```python
from build123d import *

# Parameters (mm, degrees)
F0_R     = 76.2
F0_R_2   = 1.778
F1_DEPTH = 2.921


with BuildPart() as f1:
    # F0 (on Top) → F1 (new body)
    with BuildSketch(Plane.XY):
        with Locations((76.2, 76.2)):
            Circle(F0_R)
        with Locations((35.250032, 35.250032)):
            Circle(F0_R_2, mode=Mode.SUBTRACT)
        with Locations((76.2, 8.89)):
            Circle(F0_R_2, mode=Mode.SUBTRACT)
        with Locations((117.149968, 35.250032)):
            Circle(F0_R_2, mode=Mode.SUBTRACT)
        with Locations((76.2, 66.675)):
            Circle(F0_R_2, mode=Mode.SUBTRACT)
        with Locations((8.89, 76.2)):
            Circle(F0_R_2, mode=Mode.SUBTRACT)
        with Locations((66.675, 76.2)):
            Circle(F0_R_2, mode=Mode.SUBTRACT)
        with Locations((35.250032, 117.149968)):
            Circle(F0_R_2, mode=Mode.SUBTRACT)
        with Locations((85.725, 76.2)):
            Circle(F0_R_2, mode=Mode.SUBTRACT)
        with Locations((76.2, 85.725)):
            Circle(F0_R_2, mode=Mode.SUBTRACT)
        with Locations((143.51, 76.2)):
            Circle(F0_R_2, mode=Mode.SUBTRACT)
        with Locations((76.2, 143.51)):
            Circle(F0_R_2, mode=Mode.SUBTRACT)
        with Locations((117.149968, 117.149968)):
            Circle(F0_R_2, mode=Mode.SUBTRACT)
    extrude(amount=F1_DEPTH)


solid = f1.part
```
Input: part model. Units: mm. Frame: model coordinates. Coordinates: 2 decimals unless noted, no trailing zeros. Order: outer loops, then holes, each group sorted by start corner. A loop starts at its lowest first (then second) coordinate and runs counter-clockwise, first axis right, second up. Notation, with made-up numbers: (18, 44) - (28, 44) arc R25 ccw to (28, 61) - close; hole circle Ø1 at (35.5, -6.5). An arc over 180 degrees is marked (long way). Put each result on its own line as item: value.
1. Cut plane D-D on z = 1.8. State how many separate pieces and enclosed holes the cut face has, then the cut area to 3 significant figures.
Report:
separate pieces: 1
enclosed holes: 12
area: 18,100 mm2
2. Draft query along Y for faces 1 (the face through (118.846, 35.784, 1.44)), 2 (the face through (66.28, 151.75, 1.44)), 3 (the face through (75, 77, 2.921)). Return one class per face: pulls with the +Y half, pulls with the -Y half, needs draft (parallel to the pull), parting line crosses it, or undercut.
Report:
face 1: undercut
face 2: parting line crosses it
face 3: needs draft
3. Line query: line 1 along Y through (x, z) = (76.2, 1.45); line 2 along X through (y, z) = (34, 2.4); line 3 along Y through (x, z) = (8.89, 1.95). Output: solid intervals per line, ascending.
Report:
line 1: y = 0 to 7.11, 10.67 to 64.9, 68.45 to 83.95, 87.5 to 141.73, 145.29 to 152.4
line 2: x = 12.75 to 33.99, 36.51 to 115.89, 118.41 to 139.65
line 3: y = 40.48 to 74.42, 77.98 to 111.92
4. Contact query for a flat-ended pin moving along its axis: pin 1 Ø2 at (x, y) = (76.2, 66.675) entering from +Z. Output: stop coordinate, or through.
Report:
pin 1: passes through
5. Cut plane A-A on y = 76.2. Return the cut outline in (x, z).
Report:
outline: (0, 0) - (7.11, 0) - (7.11, 2.92) - (0, 2.92) - close; (10.67, 0) - (64.9, 0) - (64.9, 2.92) - (10.67, 2.92) - close; (68.45, 0) - (83.95, 0) - (83.95, 2.92) - (68.45, 2.92) - close; (87.5, 0) - (141.73, 0) - (141.73, 2.92) - (87.5, 2.92) - close; (145.29, 0) - (152.4, 0) - (152.4, 2.92) - (145.29, 2.92) - close
6. Cut plane C-C on y = 143.51. Return the cut outline in (x, z), then the cut area to 3 significant figures.
Report:
outline: (40.48, 0) - (74.42, 0) - (74.42, 2.92) - (40.48, 2.92) - close; (77.98, 0) - (111.92, 0) - (111.92, 2.92) - (77.98, 2.92) - close
area: 198 mm2
